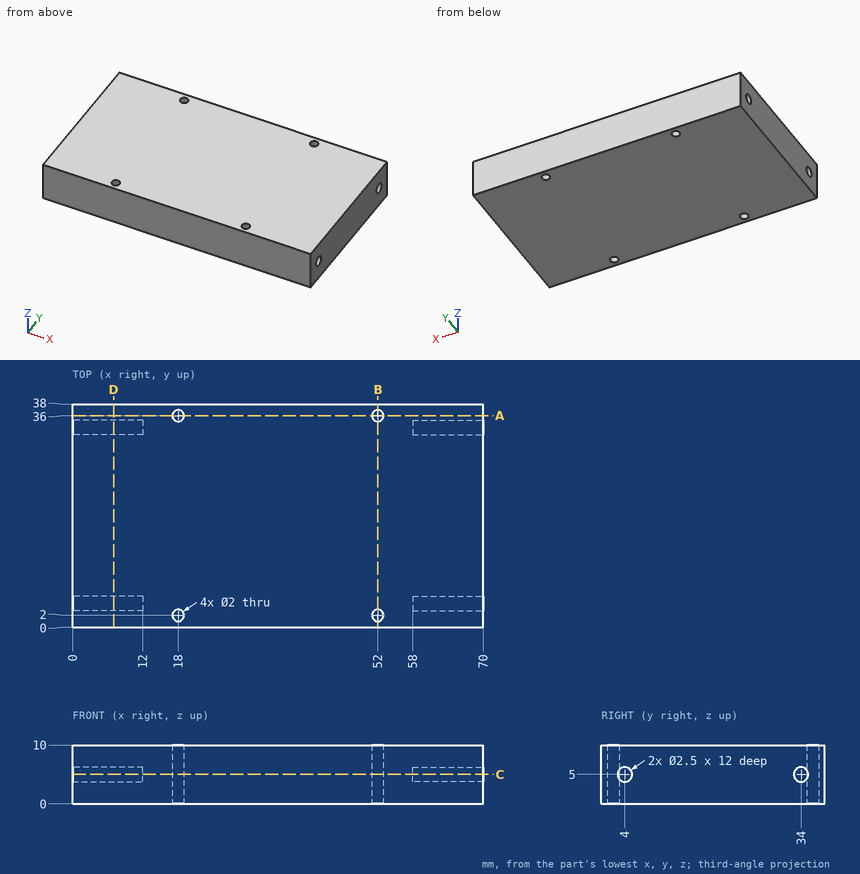
Can you work these out from the drawing? Everything is in mm from the part's minimum corner. Give positions to 0.01 mm unless a question says otherwise; leave off trailing zeros. Write each loop counter-clockwise with the first axis right and the second up, starting at its lowest first coordinate (ties: lowest second). Pieces come first, ordered by that corner, then holes. Notation, with made-up numbers: (77, -30) -> (95, -30) arc R16 ccw to (95, -16) -> close; hole circle Ø5 at (75.25, 45). An arc over 180 degrees is marked (long way). Write each question's results on one line, items separated by ' | '.
Item 1: Suppose I cut it at C-C on z = 5. Write out the boundary of the cut face in (x, y).
Output:
outline: (0, 0) -> (70, 0) -> (70, 2.75) -> (58, 2.75) -> (58, 5.25) -> (70, 5.25) -> (70, 32.75) -> (58, 32.75) -> (58, 35.25) -> (70, 35.25) -> (70, 38) -> (0, 38) -> (0, 35.25) -> (12, 35.25) -> (12, 32.75) -> (0, 32.75) -> (0, 5.25) -> (12, 5.25) -> (12, 2.75) -> (0, 2.75) -> close; hole circle Ø2 at (18, 2); hole circle Ø2 at (18, 36); hole circle Ø2 at (52, 2); hole circle Ø2 at (52, 36)
Item 2: Suppose I cut it at A-A on y = 36. Write out the boundary of the cut face in (x, z), plus the area to 3 significant figures.
Output:
outline: (0, 0) -> (17, 0) -> (17, 10) -> (0, 10) -> close; (19, 0) -> (51, 0) -> (51, 10) -> (19, 10) -> close; (53, 0) -> (70, 0) -> (70, 10) -> (53, 10) -> close | area: 660 mm^2
Item 3: For pin 1 Ø2 at (y, z) = (4, 5) entering from +X; pin 2 Ø0.8 at (y, z) = (33.5, 5) entering from -X, each with a flat end and sliding along its axis, tell me the tip position at first contact or that it passes through.
Output:
pin 1: stops at x = 58 | pin 2: stops at x = 12
Item 4: Suppose I cut it at B-B on x = 52. Write out the boundary of the cut face in (y, z).
Output:
outline: (0, 0) -> (1, 0) -> (1, 10) -> (0, 10) -> close; (3, 0) -> (35, 0) -> (35, 10) -> (3, 10) -> close; (37, 0) -> (38, 0) -> (38, 10) -> (37, 10) -> close
Item 5: If I drill on L1, parallel to Y at x = 7.5, z = 5; L2, parallel to Y at x = 18, z = 5.5; L3, parallel to X at y = 4.5, z = 4, over which ranges is the centre line in solid material (lowest first)?
Output:
L1: y = 0 to 2.75, 5.25 to 32.75, 35.25 to 38 | L2: y = 0 to 1, 3 to 35, 37 to 38 | L3: x = 12 to 58
Item 6: Suppose I cut it at D-D on x = 7. Write out the boundary of the cut face in (y, z), plus the area to 3 significant figures.
Output:
outline: (0, 0) -> (38, 0) -> (38, 10) -> (0, 10) -> close; hole circle Ø2.5 at (4, 5); hole circle Ø2.5 at (34, 5) | area: 370 mm^2
